Geometry: final body of the model. Coordinates: model frame, mm. A direction names the side the tool comes from. Coordinates: 2 decimals unless noted, no trailing zeros. Write each loop counter-clockwise with the first axis right and the second up, starting at its lowest first coordinate (ties: lowest second). Pieces come first, ordered by that corner, then holes. Notation, with made-up numbers: (-39, -31) -> (-11, -31) arc R20 cw to (-11, -4) -> close; hole circle Ø4 at (77, -15). An arc over 180 degrees is marked (long way). One line per item, written item: value. Start each with the question number.
from build123d import *

# Parameters (mm, degrees)
BOSS_EXTRUDE1_DEPTH = 40
CUT_EXTRUDE1_REACH  = 17.25
SKETCH2_R           = 4.1
SKETCH3_R           = 8
CUT_EXTRUDE2_DEPTH  = 10
FILLET1_R           = 1
CUT_EXTRUDE3_DEPTH  = 6
CUT_EXTRUDE4_REACH  = 17.5
SKETCH6_W           = 10
SKETCH6_H           = 6
SKETCH4_R           = 3.25
CUT_EXTRUDE5_DEPTH  = 3


with BuildPart() as part:
    # Sketch1 → Boss-Extrude1 (new body)
    with BuildSketch(Plane(origin=(0, 0, 0), x_dir=(0, 1, 0), z_dir=(0, 0, 1))):
        Polygon((0, 0), (0, 15.5), (11.5, 15.5), (11.5, 12.5), (15.25, 12.5), (15.25, 3), (11.5, 3), (11.5, 0), align=None)
    extrude(amount=BOSS_EXTRUDE1_DEPTH)

    # Sketch2 → Cut-Extrude1 (cut, up to next)
    with BuildSketch(Plane(origin=(0, 15.25, 0), x_dir=(-1, 0, 0), z_dir=(0, 1, 0)), mode=Mode.PRIVATE) as cut_extrude1_sk1:
        with Locations((7.75, 20)):
            Circle(SKETCH2_R)
    cut_extrude1_tool1 = extrude(cut_extrude1_sk1.sketch, amount=-CUT_EXTRUDE1_REACH, mode=Mode.PRIVATE) & part.part
    add(cut_extrude1_tool1.solids().sort_by_distance((-7.75, 15.25, 20))[0], mode=Mode.SUBTRACT)

    # Sketch3 → Cut-Extrude2 (cut)
    with BuildSketch(Plane.XZ):
        with Locations((-7.75, 20)):
            Circle(SKETCH3_R)
    extrude(amount=-CUT_EXTRUDE2_DEPTH, mode=Mode.SUBTRACT)

    # Fillet1
    fillet1_edges = [part.edges().sort_by_distance(p)[0] for p in [
        (0, 5, 18.015686517),
        (-15.5, 5, 18.015686517),
        (0, 5, 21.984313483),
        (-15.5, 5, 21.984313483),
    ]]
    fillet(fillet1_edges, radius=FILLET1_R)

    # Sketch5 → Cut-Extrude3 (cut)
    with BuildSketch(Plane.XY.offset(37)):
        Polygon((-1.976497308, 5.75), (-4.863248654, 10.75), (-10.636751346, 10.75), (-13.523502692, 5.75), (-10.636751346, 0.75), (-4.863248654, 0.75), align=None)
    extrude(amount=-CUT_EXTRUDE3_DEPTH, mode=Mode.SUBTRACT)

    # Sketch6 → Cut-Extrude4 (cut, up to next)
    with BuildSketch(Plane(origin=(-15.5, 0, 0), x_dir=(0, -1, 0), z_dir=(-1, 0, 0)), mode=Mode.PRIVATE) as cut_extrude4_sk1:
        with Locations((-5.75, 34)):
            Rectangle(SKETCH6_W, SKETCH6_H)
    cut_extrude4_tool1 = extrude(cut_extrude4_sk1.sketch, amount=-CUT_EXTRUDE4_REACH, mode=Mode.PRIVATE) & part.part
    add(cut_extrude4_tool1.solids().sort_by_distance((-15.5, 5.75, 34))[0], mode=Mode.SUBTRACT)

    # Sketch4 → Cut-Extrude5 (cut)
    with BuildSketch(Plane.XY.offset(40)):
        with Locations((-7.75, 5.75)):
            Circle(SKETCH4_R)
    extrude(amount=-CUT_EXTRUDE5_DEPTH, mode=Mode.SUBTRACT)


solid = part.part
Q1. Cut plane D-D on z = 7. Output: boundary loops of the cut face in (x, y), and give its area (3 significant figures).
Q2. Draft query along Z for faces 1 (the flat face through (-4, 10, 17)), 2 (the flat face through (-10, 10.75, 34)), 3 (the flat face through (-8, 8, 0)), 4 (the flat face through (-8, 0, 34)). Return one class per face: pulls with the +Z half, pulls with the -Z half, needs draft (parallel to the pull), parting line crosses it, or undercut.
Q3. Access query for faces 5 (the flat face through (-2, 11.5, 20)), 6 (the flat face through (-12.5, 13, 20)), 7 (the cylindrical face through (-14.869, 4.93, 25.024)). Directions: +Z, -Z, +X, -X, +Y, -Y. A direction counts if a zero-diameter tool reaches every point of the face in a straight line with its end or side. Return the directions, or none.
Q4. Cut plane A-A on z = 20. Output: boundary loops of the cut face in (x, y).
Q5. Cut plane C-C on y = 3.5. Output: boundary loops of the cut face in (x, z).
Q6. Cut plane B-B on x = -7.75. Output: boundary loops of the cut face in (y, z).
Q7. Line query: L1, parallel to Z at x = -5.5, y = 3; L2, parallel to Z at x = -13.5, y = 2.25; L3, parallel to Y at x = -7.75, z = 38.4. Output: solid intervals per line, ascending. Write a range as from..to.
Q8. First-contact query: P1, Ø8, axis at x = -6.5, z = 22.5, coming from the +Y side; P2, Ø8, axis at x = -5, z = 22.5, coming from the -Y side; P3, Ø2.5, axis at x = -14.5, z = 17.5, coming from the +Y side; P4, Ø1.1, axis at y = 13.5, z = 16.5, coming from the +X side. Flat tips, straight axial feed; report the tip coordinate or a pass-through.
Solution:
1. outline: (-15.5, 0) -> (0, 0) -> (0, 11.5) -> (-3, 11.5) -> (-3, 15.25) -> (-12.5, 15.25) -> (-12.5, 11.5) -> (-15.5, 11.5) -> close
1. area: 214 mm²
2. face 1: undercut
2. face 2: undercut
2. face 3: pulls with the -Z half
2. face 4: needs draft
3. face 5: +Z, -Z, +X, +Y
3. face 6: +Z, -Z, -X, +Y
3. face 7: -Y
4. outline: (-15.5, 10) -> (-11.85, 10) -> (-11.85, 15.25) -> (-12.5, 15.25) -> (-12.5, 11.5) -> (-15.5, 11.5) -> close; (-3.65, 10) -> (0, 10) -> (0, 11.5) -> (-3, 11.5) -> (-3, 15.25) -> (-3.65, 15.25) -> close
5. outline: (-15.5, 0) -> (0, 0) -> (0, 14.05) arc R1 ccw to (-1.75, 14.71) arc R8 cw to (-13.75, 14.71) arc R1 ccw to (-15.5, 14.05) -> close; (-15.5, 25.95) arc R1 ccw to (-13.75, 25.29) arc R8 cw to (-1.75, 25.29) arc R1 ccw to (0, 25.95) -> (0, 40) -> (-5.4, 40) -> (-5.4, 37) -> (-3.28, 37) -> (-3.28, 31) -> (-15.5, 31) -> close; (-15.5, 37) -> (-10.1, 37) -> (-10.1, 40) -> (-15.5, 40) -> close
6. outline: (0, 0) -> (15.25, 0) -> (15.25, 15.9) -> (10, 15.9) -> (10, 12) -> (0, 12) -> close; (0, 28) -> (10, 28) -> (10, 24.1) -> (15.25, 24.1) -> (15.25, 40) -> (9, 40) -> (9, 37) -> (10.75, 37) -> (10.75, 31) -> (0.75, 31) -> (0.75, 37) -> (2.5, 37) -> (2.5, 40) -> (0, 40) -> close
7. L1: 0..12.32, 27.68..31, 37..40
7. L2: 0..14.44, 25.56..31, 37..40
7. L3: 0..2.5, 9..15.25
8. P1: y = 15.25
8. P2: y = 10
8. P3: y = 11.5
8. P4: x = -3
